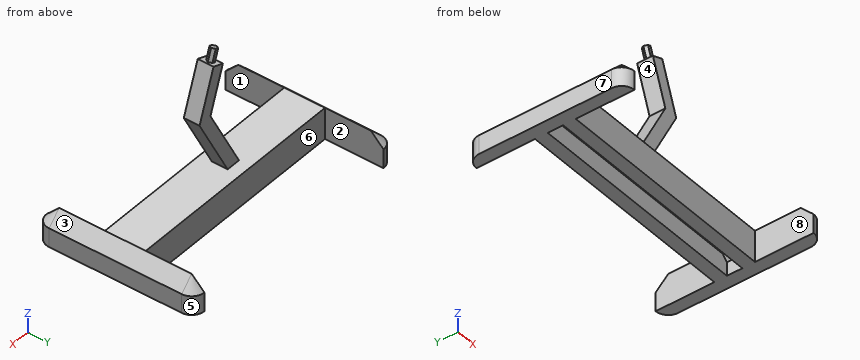
from build123d import *

# Parameters (mm, degrees)
F1_DEPTH     = 31.75
F2_DEPTH     = 3.175
F3_R         = 5.08
F4_SIZE      = 5.08
F6_DEPTH     = 5
F7_W         = 91.44
F7_H         = 18.495
F7_H_2       = 5.2874810565
F8_DEPTH     = 12.701
F9_T         = 5.08
F9_T3_DEPTH  = 22.86
F9_T5_DEPTH  = 16.51
F9_T7_DEPTH  = 15.9213350007
F9_T9_DEPTH  = 11.66
F9_T11_DEPTH = 11.5016876048
F9_T13_DEPTH = 11.66
F9_T15_DEPTH = 11.66
F9_T17_DEPTH = 11.5016876048
F9_T19_DEPTH = 11.66


# Not quite as in the source:
# - a shell that OpenCascade refuses in one call is made with other operations: the cavity is built on its own and cut out


with BuildPart() as f1:
    # F0 (on Front) → F1 (new body, symmetric)
    with BuildSketch(Plane.XZ):
        Polygon((50.8, -6.35), (50.8, 6.35), (-2.4423953146, 6.35), (-8.2037303153, 6.35), (-50.8, 6.35), (-50.8, -6.35), align=None)
    extrude(amount=F1_DEPTH, both=True)

    # F0 (on Front) → F2 (join, symmetric)
    with BuildSketch(Plane.XZ):
        Polygon((-8.2037303153, 6.35), (-2.4423953146, 6.35), (11.905341187, 33.1679385818), (4.7710500911, 52.6789357495), (0, 50.9343780577), (6.3533243835, 33.5591837482), align=None)
    extrude(amount=F2_DEPTH, both=True)

    # F3
    f3_edges = [f1.edges().sort_by_distance(p)[0] for p in [
        (-50.8, -31.75, 0),
        (50.8, -31.75, 0),
        (50.8, 31.75, 0),
        (-50.8, 31.75, 0),
    ]]
    fillet(f3_edges, radius=F3_R)

    # F4
    f4_edges = [f1.edges().sort_by_distance(p)[0] for p in [
        (50.8, 0, 6.35),
    ]]
    chamfer(f4_edges, length=F4_SIZE)

    # F5 (on face) → F6 (join)
    with BuildSketch(Plane(origin=(-16.4279316214, 0, 44.9274248875), x_dir=(0.9391830795, 0, 0.3434168651), z_dir=(-0.3434168651, 0, 0.9391830795))):
        Polygon((20.5937571299, 1.25), (19.2520695251, 1.25), (18.4229133275, 0), (19.2520695251, -1.25), (20.5937571299, -1.25), (21.4229133275, 0), align=None)
    extrude(amount=F6_DEPTH)

    # F7 (on face) → F8 (cut, through all)
    with BuildSketch(Plane.XY.offset(6.35)):
        with Locations((0, -17.4225)):
            Rectangle(F7_W, F7_H)
        with Locations((0, 17.4225)):
            Rectangle(F7_W, F7_H)
        with Locations((0, -29.3137405282)):
            Rectangle(F7_W, F7_H_2)
        with Locations((0, 29.3137405282)):
            Rectangle(F7_W, F7_H_2)
    extrude(amount=-F8_DEPTH, mode=Mode.SUBTRACT)

    # F9: shell of thickness 5.08, made by hand


with BuildPart() as f9_core1:
    # F9_t2: copy of F1
    add(f1.part)

    # the walls: a layer under each face that stays
    f9_faces = [f9_core1.faces().sort_by_distance(p)[0] for p in [
        (50.8, 0, -2.54),
        (48.26, 0, 3.81),
        (47.5160512242, 28.4660512242, 3.81),
        (45.72, 19.9625, 0),
        (0, 0, 6.35),
        (45.72, -19.9625, 0),
        (47.5160512242, -28.4660512242, 3.81),
        (-50.8, 0, -2.54),
        (-45.72, -19.9625, 0),
        (0, -8.175, 0),
        (0, 8.175, 0),
        (-45.72, 19.9625, 0),
        (-48.26, 0, 3.81),
        (-0.9252029659, 0, 19.9545918741),
        (8.55382927, 3.175, 29.5144678748),
        (8.55382927, -3.175, 29.5144678748),
        (4.7314729362, 0, 19.7589692909),
        (-47.5160512242, 28.4660512242, 3.81),
        (-47.5160512242, -28.4660512242, 3.81),
        (3.1766621917, 0, 42.246780903),
        (8.3381956391, 0, 42.9234371656),
        (3.975875076, 2.1166666667, 52.3881761342),
        (2.444199191, 0.625, 54.4899992105),
        (1.4247893073, 1.25, 54.1172470239),
        (0.4053794236, 0.625, 53.7444948373),
        (0.4053794236, -0.625, 53.7444948373),
        (1.4247893073, -1.25, 54.1172470239),
        (2.444199191, -0.625, 54.4899992105),
        (0.5662471447, 0, 56.4652047226),
    ]]
    thicken(f9_faces, amount=-F9_T, mode=Mode.SUBTRACT)

    # F9_s4 → F9_t3 (cut)
    with BuildSketch(Plane.XY.offset(-11.43)):
        Polygon((45.6692, 8.2258), (50.8, 8.175), (50.8, 3.095), (45.72, 3.095), align=None)
        Polygon((45.6692, -8.2258), (50.8, -8.175), (50.8, -3.095), (45.72, -3.095), align=None)
        Polygon((-45.6692, -8.2258), (-50.8, -8.175), (-50.8, -3.095), (-45.72, -3.095), align=None)
        Polygon((-45.6692, 8.2258), (-45.72, 3.095), (-50.8, 3.095), (-50.8, 8.175), align=None)
    extrude(amount=F9_T3_DEPTH, mode=Mode.SUBTRACT)

    # F9_s6 → F9_t5 (cut)
    with BuildSketch(Plane.XZ.offset(-8.255)):
        Polygon((-8.2485227119, 6.424764165), (-8.2037303153, 1.27), (-5.1602217701, 1.27), (-3.7244906507, 3.9535835029), align=None)
        Polygon((-2.3976029179, 6.376835835), (-2.4423953146, 1.27), (-10.9215566565, 1.27), (-6.9216349791, 8.7464164971), align=None)
        Polygon((6.2608214864, 33.5657023365), (10.832564048, 31.1627672512), (11.9053411319, 33.1679385857), (11.1243744273, 35.3037414227), align=None)
    extrude(amount=F9_T5_DEPTH, mode=Mode.SUBTRACT)

    # F9_s8 → F9_t7 (cut)
    with BuildSketch(Plane.YZ.offset(-13.2837303153)):
        Polygon((3.2258, 6.4008), (3.175, 1.27), (-1.905, 1.27), (-1.905, 6.35), align=None)
        Polygon((-3.2258, 6.4008), (-3.175, 1.27), (1.905, 1.27), (1.905, 6.35), align=None)
    extrude(amount=F9_T7_DEPTH, mode=Mode.SUBTRACT)

    # F9_s10 → F9_t9 (cut)
    with BuildSketch(Plane(origin=(8.7850864423, -14.1016340866, 3.2123096243), x_dir=(-0.8487666121, -0.5287676599, 0), z_dir=(-0.5191529807, 0.8333333333, -0.1898308147))):
        Polygon((-3.1675232496, 51.0265185517), (-4.6144586839, 46.1037076546), (0.2449508944, 44.6229853476), (1.7256732014, 49.4823949258), align=None)
    extrude(amount=F9_T9_DEPTH, mode=Mode.SUBTRACT)

    # F9_s12 → F9_t11 (cut)
    with BuildSketch(Plane(origin=(24.1123582833, 0, 8.8168011877), x_dir=(0, 1, 0), z_dir=(-0.9391830795, 0, -0.3434168651))):
        Polygon((1.3008, -47.8875060361), (1.25, -42.7567060361), (-3.83, -42.7567060361), (-3.83, -47.8367060361), align=None)
    extrude(amount=F9_T11_DEPTH, mode=Mode.SUBTRACT)

    # F9_s14 → F9_t13 (cut)
    with BuildSketch(Plane(origin=(8.7028980905, 13.9697070906, 3.1822570534), x_dir=(0.8487666121, -0.5287676599, 0), z_dir=(-0.5191529807, -0.8333333333, -0.1898308147))):
        Polygon((0.6788933364, 50.2682021828), (2.2230169623, 45.3750057318), (7.0824265406, 46.8557280388), (5.6017042336, 51.7151376171), align=None)
    extrude(amount=F9_T13_DEPTH, mode=Mode.SUBTRACT)

    # F9_s16 → F9_t15 (cut)
    with BuildSketch(Plane(origin=(2.6495743357, -4.253040424, 0.9688297542), x_dir=(0.8487666121, 0.5287676599, 0), z_dir=(0.5191529807, -0.8333333333, 0.1898308147))):
        Polygon((0.6788933364, 50.2682021828), (2.2230169623, 45.3750057318), (7.0824265406, 46.8557280388), (5.6017042336, 51.7151376171), align=None)
    extrude(amount=F9_T15_DEPTH, mode=Mode.SUBTRACT)

    # F9_s18 → F9_t17 (cut)
    with BuildSketch(Plane(origin=(13.3101678993, 0, 4.8669276876), x_dir=(0, 1, 0), z_dir=(0.9391830795, 0, 0.3434168651))):
        Polygon((-1.3008, 47.8875060361), (-1.25, 42.7567060361), (3.83, 42.7567060361), (3.83, 47.8367060361), align=None)
    extrude(amount=F9_T17_DEPTH, mode=Mode.SUBTRACT)

    # F9_s20 → F9_t19 (cut)
    with BuildSketch(Plane(origin=(2.7317626875, 4.38496742, 0.9988823252), x_dir=(-0.8487666121, 0.5287676599, 0), z_dir=(0.5191529807, 0.8333333333, 0.1898308147))):
        Polygon((-3.1675232496, 51.0265185517), (-4.6144586839, 46.1037076546), (0.2449508944, 44.6229853476), (1.7256732014, 49.4823949258), align=None)
    extrude(amount=F9_T19_DEPTH, mode=Mode.SUBTRACT)


with BuildPart() as f1_1:
    add(f1.part)

    # what is left inside the walls is the cavity
    f9_cavity = [f9_core1.part.solids().sort_by_distance(p)[0] for p in [
        (0, 3.0442, -3.81),
    ]]
    add(f9_cavity, mode=Mode.SUBTRACT)


solid = f1_1.part
CAD build for the part. Positions are in the model's coordinates, mm. Face numbers are marked on the shaded views. A direction names the side the tool comes from. Round coordinates to 2 decimals unless told otherwise and drop trailing zeros. Order: outer loops, then holes, each group sorted by start corner. A loop starts at its lowest first (then second) coordinate and runs counter-clockwise, first axis right, second up. Notation, with made-up numbers: M 26.25,-29.5 L 50.25,-29.5 A29 cw 50.25,2.5 Z; hole C 74.5,39.5 d3. An arc over 180 degrees is marked long. Use one line per item in the form item = value.
Q1. Saw through at B-B on x = 7.5. Give the cut face in (y, z) (3 decimals), then the cut area to 3 significant figures.
Recorded:
outline = M -8.175,-6.35 L -3.095,-6.35 L -3.095,1.27 L 3.095,1.27 L 3.095,-6.35 L 8.175,-6.35 L 8.175,6.35 L -8.175,6.35 Z; M -3.175,24.934 L 3.175,24.934 L 3.175,45.216 L -3.175,45.216 Z
area = 289 mm^2
Q2. Saw through at D-D on z = 24. Give the cut face in (x, y) (3 decimals).
Recorded:
outline = M 1.239,-3.175 L 7,-3.175 L 7,3.175 L 1.239,3.175 Z
Q3. Saw through at C-C on z = 39. Give the cut face in (x, y) (3 decimals).
Recorded:
outline = M 4.364,-3.175 L 9.773,-3.175 L 9.773,3.175 L 4.364,3.175 Z
Q4. Probe L1, parallel to Y at x = -35, z = -2 (3 decimals); L2, parallel to Z at x = 17, y = -5.5; L3, parallel to Y at x = 41, z = 4 (3 decimals). List the from-to ranges inside material, lowest first.
Recorded:
L1 = -8.175 to -3.095, 3.095 to 8.175
L2 = -6.35 to 6.35
L3 = -8.175 to 8.175
Q5. Saw through at A-A on y = 25. Give the cut face in (x, z), then the cut area to 3 significant figures.
Recorded:
outline = M -50.8,-6.35 L -45.72,-6.35 L -45.72,6.35 L -50.8,1.27 Z; M 45.72,-6.35 L 50.8,-6.35 L 50.8,1.27 L 45.72,6.35 Z
area = 103 mm^2
Q6. Which spindle directions (+Z, -Z, +X, -X, +Y, -Y) get a long thin tool onto all of the face, cutting with end or side? Do the marked faces 1, 2, 3 and 4. Say none if no direction does.
Recorded:
face_1 = +Z, -Z, -Y
face_2 = +Z, -Z, +Y
face_3 = +Z, +X, +Y, -Y
face_4 = -X, +Y, -Y
Q7. Two-plate mould, pull along X, no slides. Class the marked faces 5, 6, 7 and 8: +X half, -X half, draft (parallel to the pull), parting line (faces both ways), or undercut.
Recorded:
face_5 = +X half
face_6 = undercut
face_7 = -X half
face_8 = undercut
Q8. Flat gauge pins, fed straight in: P1, Ø12, axis at x = -4, z = 48.5, coming from the -Y side (3 decimals); P2, Ø12, axis at x = 23, z = 33.5, coming from the -Y side; P3, Ø4, axis at x = 11, z = -2.5, coming from the -Y side (3 decimals); P4, Ø0.9, axis at x = 1.5, z = 54.5, coming from the +Y side. Where does each tip first touch, or does it go through?
Recorded:
P1 = -3.175
P2 = through
P3 = -8.175
P4 = 1.25
